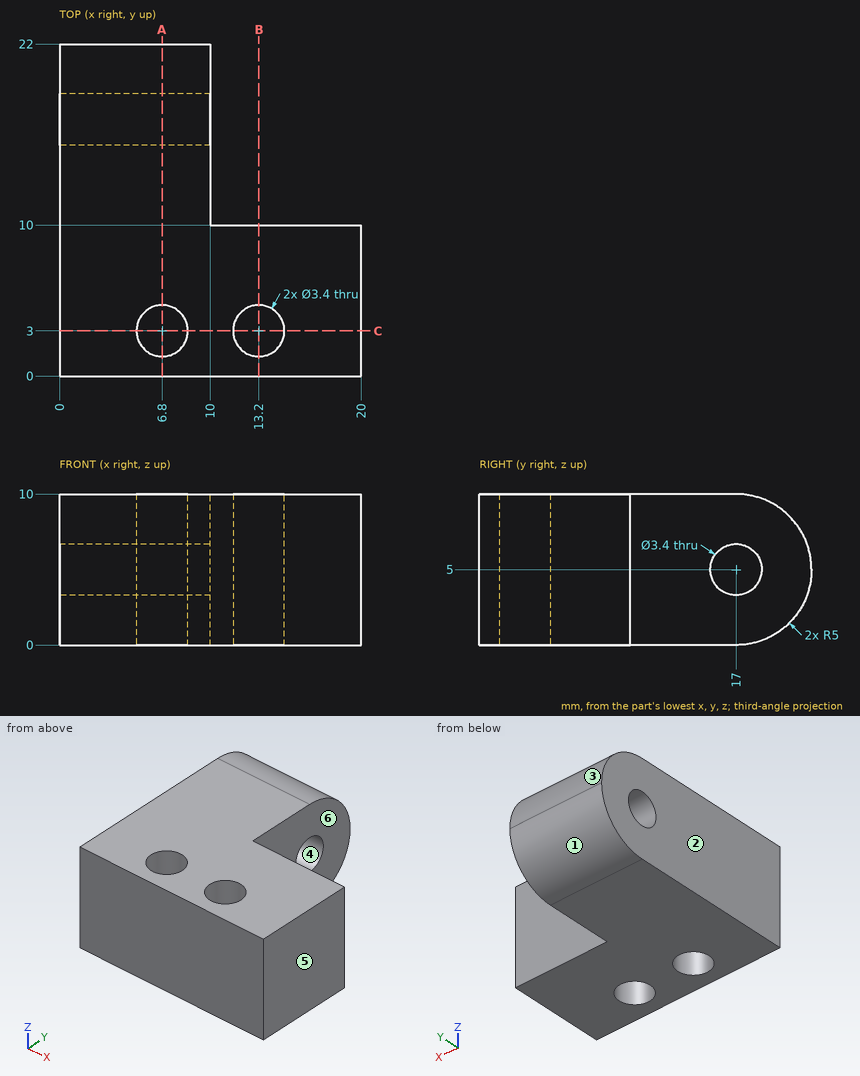
Design review of the part shown in the three views and the two pictorial views. Dimensions are in mm from the part's minimum x, y and z. A direction names the side the tool comes from. Coordinates: 2 decimals unless noted, no trailing zeros. Write each loop counter-clockwise with the first axis right and the second up, starting at its lowest first coordinate (ties: lowest second). Pieces come first, ordered by that corner, then holes.
1) Machinability: for the marked faces 5 and 6, which of the approach directions +Z, -Z, +X, -X, +Y, -Y give a long, thin tool a straight path to every point of the face, cutting with its end or side? Answer none if there is none.
2) The part is to be moulded in two halves that separate along Z. For the marked faces 1, 2, 3 and 4, say which applies: pulls with the +Z half, pulls with the -Z half, needs draft (parallel to the pull), parting line crosses it, or undercut.
3) To check wall thickness, follow probe 1 along Y at (x, z) = (13.2, 7); probe 2 along Y at (x, z) = (6.8, 4.25) (1 decimal); probe 3 along Y at (x, z) = (5.25, 5) (1 decimal). State the ranges of each line that lie inside material, in increasing order.
4) We need section A-A on x = 6.8. Count the separate pieces of the cut face and the enclosed holes in it, then the cut area to 3 significant figures.
5) We need section C-C on y = 3. State the section outline as (x, z) points, then the cut area to 3 significant figures.
6) We need section B-B on x = 13.2. State the section outline as (y, z) points.
7) Clearance check with flat-ended pins moving along their axes: pin 1 Ø4 at (y, z) = (5, 2) entering from -X; pin 2 Ø5 at (y, z) = (17.5, 5.5) entering from +X; pin 3 Ø2.5 at (x, y) = (13.2, 3) entering from -Z; pin 4 Ø1.5 at (x, z) = (18, 2) entering from +Y. State where each tip first meets the part, or that it passes through.
Answer list:
1. face 5: +Z, -Z, +X, +Y, -Y
1. face 6: +Z, -Z, +X, +Y
2. face 1: pulls with the -Z half
2. face 2: needs draft
2. face 3: pulls with the +Z half
2. face 4: undercut
3. probe 1: y = 0 to 1.3, 4.7 to 10
3. probe 2: y = 0 to 1.3, 4.7 to 15.5, 18.5 to 21.9
3. probe 3: y = 0 to 2.3, 3.7 to 15.3, 18.7 to 22
4. separate pieces: 2
4. enclosed holes: 1
4. area: 166 mm2
5. outline: (0, 0) - (5.1, 0) - (5.1, 10) - (0, 10) - close; (8.5, 0) - (11.5, 0) - (11.5, 10) - (8.5, 10) - close; (14.9, 0) - (20, 0) - (20, 10) - (14.9, 10) - close
5. area: 132 mm2
6. outline: (0, 0) - (1.3, 0) - (1.3, 10) - (0, 10) - close; (4.7, 0) - (10, 0) - (10, 10) - (4.7, 10) - close
7. pin 1: stops at x = 0
7. pin 2: stops at x = 10
7. pin 3: passes through
7. pin 4: stops at y = 10
